Verification items for this drawing (mm, ordinates from the low corner). A direction names the side the tool comes from. Round coordinates to 2 decimals unless told otherwise and drop trailing zeros. Loops run counter-clockwise (first coordinate to the right, second up) from the corner with the lowest first, then second, coordinate; pieces in that order, holes last. Notation, with made-up numbers: (68.25, -25) - (110.25, -25) arc R9 ccw to (110.25, -15) - close; hole circle Ø8 at (21.5, -19). An arc over 180 degrees is marked (long way). Put each result on its own line as item: value.
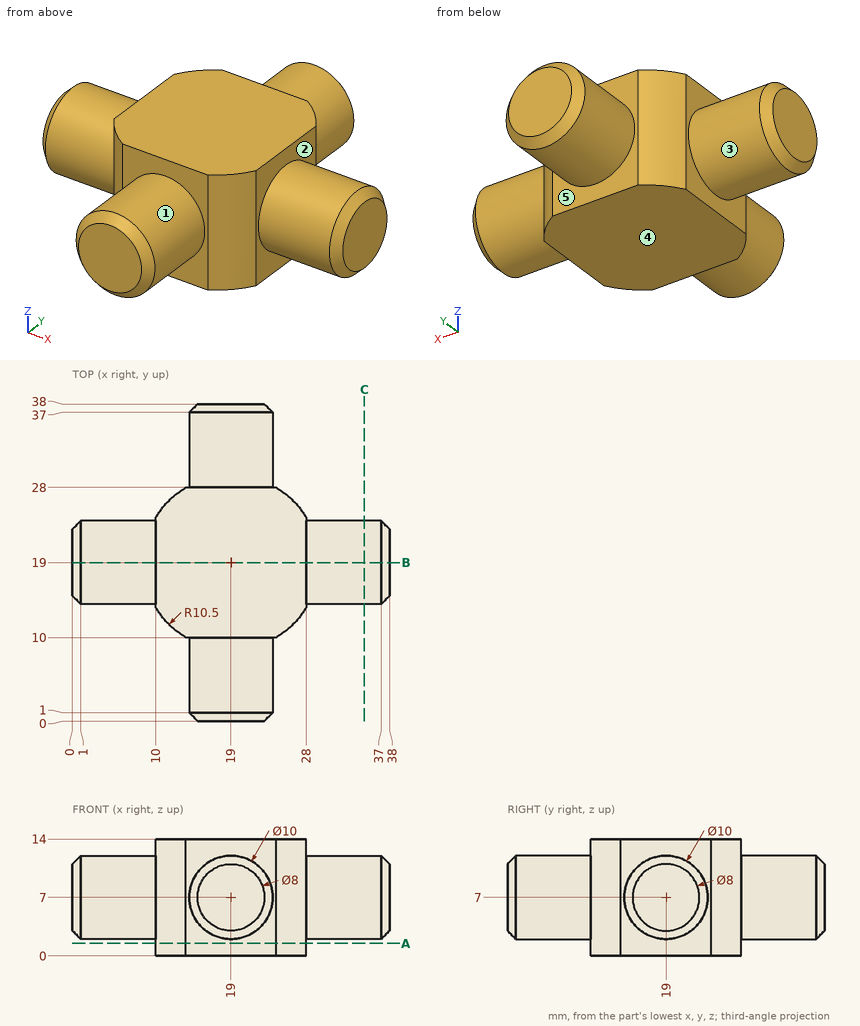
Item 1: Section check B-B on y = 19. Enter the section's corners in (x, z).
Filled sheet:
outline: (0, 3) - (1, 2) - (10, 2) - (10, 0) - (28, 0) - (28, 2) - (37, 2) - (38, 3) - (38, 11) - (37, 12) - (28, 12) - (28, 14) - (10, 14) - (10, 12) - (1, 12) - (0, 11) - close
Item 2: Go/stop test with flat-tipped pins: pin 1 (1 mm diameter, centred on x = 6, y = 21.5, fed in from +Z); pin 2 (1.5 mm diameter, centred on x = 14.5, z = 4, fed in from +Y); pin 3 (1 mm diameter, centred on y = 33, z = 9, fed in from -X). Record where each tip stops, or that it passes through.
Filled sheet:
pin 1: z = 11.58
pin 2: y = 37.34
pin 3: x = 14.23
Item 3: Tool access check on the marked faces 1, 2, 3, 4 and 5. Record the directions out of +Z, -Z, +X, -X, +Y, -Y that give a thin tool (end or side, any length) a straight path to the whole face; none if there is none.
Filled sheet:
face 1: -Y
face 2: +X
face 3: -X
face 4: -Z, +X, -X, +Y, -Y
face 5: +Y
Item 4: Section check A-A on z = 1.5. Enter the section's corners in (x, y).
Filled sheet:
outline: (10, 13.59) arc R10.5 ccw to (13.59, 10) - (24.41, 10) arc R10.5 ccw to (28, 13.59) - (28, 24.41) arc R10.5 ccw to (24.41, 28) - (13.59, 28) arc R10.5 ccw to (10, 24.41) - close
Item 5: Section check C-C on x = 35. Enter the section's corners in (y, z), then the cut area to 3 significant figures.
Filled sheet:
outline: circle Ø10 at (19, 7)
area: 78.5 mm²
Item 6: Thickness scan on line 1 (Y direction, x = 23, z = 3.75); line 2 (X direction, y = 6.5, z = 6.75); line 3 (Y direction, x = 2, z = 4). Record the ranges inside material, lowest first. Write a range as from..to.
Filled sheet:
line 1: 10..28
line 2: 14.01..23.99
line 3: 15..23
